Geometry check sheet. Reference: the model listing, model coordinates, mm. Coordinates: 2 decimals unless noted, no trailing zeros. Order: outer loops, then holes, each group sorted by start corner. A loop starts at its lowest first (then second) coordinate and runs counter-clockwise, first axis right, second up. Notation, with made-up numbers: (-0.75, -1) - (36.25, -1) arc R31 ccw to (36.25, 31) - close; hole circle Ø10 at (38, 9.25). An arc over 180 degrees is marked (long way). One line per item, written item: value. Start each with the question number.
Autodesk Inventor part; units mm, degrees
ref_plane "YZ Plane" through (0, 0, 0) normal (1, 0, 0) x (0, 1, 0)
ref_plane "XZ Plane" through (0, 0, 0) normal (0, 1, 0) x (-1, 0, 0)
ref_plane "XY Plane" through (0, 0, 0) normal (0, 0, 1) x (1, 0, 0)
sketch "Sketch1" plane through (0, 0, 0) normal (0, 0, 1) x (1, 0, 0)
  line L0 (0, 0) -> (200, 0) construction
  arc A0 (200, 0) -> (0, 0) centre (100, -2022.5294) ccw
  line L1 (200, 0) -> (226.0472, 147.7212)
  line L2 (200, 0) -> (350, 0) construction
  line L3 (100, 2.4706) -> (100, 110.946)
  line L4 (0, 0) -> (-26.0472, 147.7212)
  arc A1 (226.0472, 147.7212) -> (-26.0472, 147.7212) centre (100, -252.9184) ccw
  dimension "d4" = 2025
  dimension "d5" = 150
  dimension "d6" = 80
  dimension "d7" = 420
  dimension "d20" = 200
extrude "Plate1" add sketch "Sketch1" along normal blind 6
sketch "Sketch2" plane through (0, 0, 6) normal (0, 0, 1) x (1, 0, 0)
  arc A0 (200, 0) -> (0, 0) centre (100, -2022.5294) ccw
  line L0 (100, 2.4706) -> (100, 167.0816)
  arc A1 (226.0472, 147.7212) -> (-26.0472, 147.7212) centre (100, -252.9184) ccw
  arc A2 (100, 2.4706) -> (0, 0) centre (100, -2022.5294) ccw
  arc A3 (100, 167.0816) -> (-26.0472, 147.7212) centre (100, -252.9184) ccw
  line L1 (45.7974, 79.0021) -> (15.7974, 79.0021) construction
  line L2 (45.7974, 84.2521) -> (15.7974, 84.2521)
  line L3 (15.7974, 73.7521) -> (45.7974, 73.7521)
  arc A4 (45.7974, 73.7521) -> (45.7974, 84.2521) centre (45.7974, 79.0021) ccw
  arc A5 (15.7974, 84.2521) -> (15.7974, 73.7521) centre (15.7974, 79.0021) ccw
  line L4 (30.7974, 79.0021) -> (27.8022, 113.8737)
  line L5 (30.7974, 79.0021) -> (33.7926, 44.1305)
  line L6 (18.7926, 44.1305) -> (48.7926, 44.1305) construction
  line L7 (18.7926, 38.8805) -> (48.7926, 38.8805)
  line L8 (48.7926, 49.3805) -> (18.7926, 49.3805)
  arc A6 (18.7926, 49.3805) -> (18.7926, 38.8805) centre (18.7926, 44.1305) ccw
  arc A7 (48.7926, 38.8805) -> (48.7926, 49.3805) centre (48.7926, 44.1305) ccw
  line L9 (33.7926, 44.1305) -> (63.7926, 44.1305) construction
  line L10 (12.8022, 113.8737) -> (42.8022, 113.8737) construction
  line L11 (12.8022, 108.6237) -> (42.8022, 108.6237)
  line L12 (42.8022, 119.1237) -> (12.8022, 119.1237)
  arc A8 (12.8022, 119.1237) -> (12.8022, 108.6237) centre (12.8022, 113.8737) ccw
  arc A9 (42.8022, 108.6237) -> (42.8022, 119.1237) centre (42.8022, 113.8737) ccw
  line L13 (154.2026, 79.0021) -> (184.2026, 79.0021) construction
  line L14 (154.2026, 84.2521) -> (184.2026, 84.2521)
  line L15 (184.2026, 73.7521) -> (154.2026, 73.7521)
  arc A10 (154.2026, 84.2521) -> (154.2026, 73.7521) centre (154.2026, 79.0021) ccw
  arc A11 (184.2026, 73.7521) -> (184.2026, 84.2521) centre (184.2026, 79.0021) ccw
  line L16 (169.2026, 79.0021) -> (172.1978, 113.8737)
  line L17 (169.2026, 79.0021) -> (166.2074, 44.1305)
  line L18 (181.2074, 44.1305) -> (151.2074, 44.1305) construction
  line L19 (181.2074, 38.8805) -> (151.2074, 38.8805)
  line L20 (151.2074, 49.3805) -> (181.2074, 49.3805)
  arc A12 (181.2074, 38.8805) -> (181.2074, 49.3805) centre (181.2074, 44.1305) ccw
  arc A13 (151.2074, 49.3805) -> (151.2074, 38.8805) centre (151.2074, 44.1305) ccw
  line L21 (187.1978, 113.8737) -> (157.1978, 113.8737) construction
  line L22 (187.1978, 108.6237) -> (157.1978, 108.6237)
  line L23 (157.1978, 119.1237) -> (187.1978, 119.1237)
  arc A14 (187.1978, 108.6237) -> (187.1978, 119.1237) centre (187.1978, 113.8737) ccw
  arc A15 (157.1978, 119.1237) -> (157.1978, 108.6237) centre (157.1978, 113.8737) ccw
  dimension "d9" = 15
  dimension "d10" = 10.5
  dimension "d11" = 35
  dimension "d12" = 35
  dimension "d13" = 15
  dimension "d14" = 0
  dimension "d15" = 10.5
  dimension "d16" = 15
  dimension "d17" = 10.5
extrude "Cut1" cut sketch "Sketch2" against normal blind 6
fillet "Fillet1" radius 10 1 edges at (100, 2.4706, 0)
equation "\"d18\" = Thickness"
equation "\"d8\" = Thickness"
equation "\"BendRadius\" = Thickness"
equation "\"BendReliefWidth\" = Thickness"
equation "\"BendReliefDepth\" = 0.5 * Thickness"
equation "\"CornerReliefSize\" = 4 * Thickness"
equation "\"MinimumRemnant\" = 2 * Thickness"
equation "\"TransitionRadius\" = BendRadius"
equation "\"JacobiRadiusSize\" = BendRadius"
equation "\"GapSize\" = Thickness"
properties part number "Double Shear Plate"
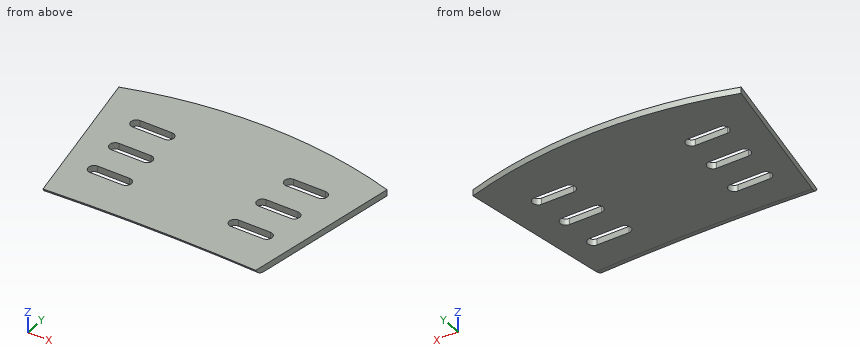
Q1. Cross-section at B-B, the plane y = 35.5. Enter the section's corners in (x, z), and give its area (3 significant figures).
Q2. Cross-section at D-D, the plane y = 55. Enter the section's corners in (x, z), and give its area (3 significant figures).
Q3. Gauge pin test, flat ends, axial feed: P1, Ø3, axis at x = 161, z = 2, coming from the -Y side; P2, Ø1.5, axis at y = 96, z = 5, coming from the +X side; P3, Ø3, axis at x = 167, z = 3, coming from the +Y side; P4, Ø8, axis at x = 17.5, y = 101, coming from the -Z side. Record the tip position at first contact, or that the pin passes through.
Q4. Material ranges on probe 1 along X at (y, z) = (39.5, 3); probe 2 along X at (y, z) = (48, 0.5); probe 3 along Y at (x, z) = (155, 3), recorded low to high.
Q5. Cross-section at C-C, the plane x = 34. Count the separate pieces of the cut face and the enclosed holes in it, and give its area (3 significant figures).
Q6. Cross-section at A-A, the plane z = 1. Enter the section's corners in (x, y), and give its area (3 significant figures).
Check result:
1. outline: (-6.26, 0) - (206.26, 0) - (206.26, 6) - (-6.26, 6) - close
1. area: 1,280 mm2
2. outline: (-9.7, 0) - (209.7, 0) - (209.7, 6) - (-9.7, 6) - close
2. area: 1,320 mm2
3. P1: stops at y = 3.12
3. P2: stops at x = 217.06
3. P3: stops at y = 161.94
3. P4: stops at z = 0
4. probe 1: x = -6.96 to 16.32, 51.27 to 148.73, 183.68 to 206.96
4. probe 2: x = -8.46 to 15.24, 52.34 to 147.66, 184.76 to 208.46
4. probe 3: y = 3.75 to 38.88, 49.38 to 73.75, 84.25 to 109.11, 118.64 to 163.46
5. separate pieces: 4
5. enclosed holes: 0
5. area: 758 mm2
6. outline: (-26.05, 147.72) - (-0.84, 4.77) arc R2029.81 cw to (200.84, 4.77) - (226.05, 147.72) arc R420 ccw to start; hole (12.8, 108.62) - (42.8, 108.62) arc R5.25 ccw to (42.8, 119.12) - (12.8, 119.12) arc R5.25 ccw to start; hole (15.8, 73.75) - (45.8, 73.75) arc R5.25 ccw to (45.8, 84.25) - (15.8, 84.25) arc R5.25 ccw to start; hole (18.79, 38.88) - (48.79, 38.88) arc R5.25 ccw to (48.79, 49.38) - (18.79, 49.38) arc R5.25 ccw to start; hole (151.21, 38.88) - (181.21, 38.88) arc R5.25 ccw to (181.21, 49.38) - (151.21, 49.38) arc R5.25 ccw to start; hole (154.2, 73.75) - (184.2, 73.75) arc R5.25 ccw to (184.2, 84.25) - (154.2, 84.25) arc R5.25 ccw to start; hole (157.2, 108.62) - (187.2, 108.62) arc R5.25 ccw to (187.2, 119.12) - (157.2, 119.12) arc R5.25 ccw to start
6. area: 33,000 mm2
